```python
from build123d import *

# Parameters (mm, degrees)
SKETCH_R        = 12.5
PAD_DEPTH       = 30
SKETCH001_R     = 5
POCKET_DEPTH    = 10
SKETCH002_R     = 4
POCKET001_DEPTH = 10


with BuildPart() as part:
    # Sketch → Pad (new body)
    with BuildSketch(Plane.XZ):
        Circle(SKETCH_R)
    extrude(amount=PAD_DEPTH)

    # Sketch001 (on Face3 of Pad) → Pocket (cut)
    with BuildSketch(Plane.XZ.offset(30)):
        Circle(SKETCH001_R)
    extrude(amount=-POCKET_DEPTH, mode=Mode.SUBTRACT)

    # Sketch002 (on Face2 of Pocket) → Pocket001 (cut)
    with BuildSketch(Plane(origin=(0, 0, 0), x_dir=(1, 0, 0), z_dir=(0, 1, 0))):
        Circle(SKETCH002_R)
    extrude(amount=-POCKET001_DEPTH, mode=Mode.SUBTRACT)


solid = part.part
```
Model file for the job. Use its own axes, mm. A direction names the side the tool comes from. Coordinates: 2 decimals unless noted, no trailing zeros. Write each loop counter-clockwise with the first axis right and the second up, starting at its lowest first coordinate (ties: lowest second). Pieces come first, ordered by that corner, then holes. Notation, with made-up numbers: (30, 87.25) - (85, 87.25) arc R31 cw to (85, 124.25) - close; hole circle Ø10 at (-11, 31.5). An arc over 180 degrees is marked (long way). One line per item, written item: value. Start each with the question number.
1. Flat gauge pins, fed straight in: pin 1 (1 mm diameter, centred on x = 3, z = -1.5, fed in from +Y); pin 2 (2 mm diameter, centred on x = -5, y = -15, fed in from +Z); pin 3 (2 mm diameter, centred on y = -25, z = -9, fed in from -X). Where does each tip first touch, or does it go through?
2. Probe line 1 (Z direction, x = 0, y = -2.25); line 2 (Z direction, x = 0, y = -24.75); line 3 (X direction, y = -8.25, z = -2.75). List the from-to ranges inside material, lowest first. Write a range as from..to.
3. Slice it at C-C (y = -7.75). Write the cut outline in (x, z).
4. Mould opens along Z. For faces 4 (the cylindrical face through (11.923, -14.79, 3.755)), 5 (the flat face through (-3, 0, 3)), 6 (the flat face through (0, -20, 0)) say: released by +Z, released by -Z, zero draft, split by the parting line, or undercut.
5. Tool access for faces 1 (the cylindrical face through (-0.867, -4.93, 3.905)), 2 (the flat face through (-0.2, -30, -5.4)), 3 (the cylindrical face through (-1.08, -25.07, -4.88)): list every direction of +Z, -Z, +X, -X, +Y, -Y with a clear straight run to the whole face (end or side of a thin tool).
6. Slice it at B-B (x = 0). Write the cut outline in (y, z), plus the area to 3 significant figures.
7. Slice it at D-D (y = -12.5). Write the cut outline in (x, z), plus the area to 3 significant figures.
8. Slice it at A-A (z = 0). Write the cut outline in (x, y).
Answers below:
1. pin 1: stops at y = -10
1. pin 2: stops at z = 11.84
1. pin 3: stops at x = -9.6
2. line 1: z = -12.5..-4, 4..12.5
2. line 2: z = -12.5..-5, 5..12.5
2. line 3: x = -12.19..-2.9, 2.9..12.19
3. outline: circle Ø25 at (0, 0); hole circle Ø8 at (0, 0)
4. face 4: split by the parting line
4. face 5: zero draft
4. face 6: undercut
5. face 1: +Y
5. face 2: +Z, -Z, +X, -X, -Y
5. face 3: -Y
6. outline: (-30, -12.5) - (0, -12.5) - (0, -4) - (-10, -4) - (-10, 4) - (0, 4) - (0, 12.5) - (-30, 12.5) - (-30, 5) - (-20, 5) - (-20, -5) - (-30, -5) - close
6. area: 570 mm^2
7. outline: circle Ø25 at (0, 0)
7. area: 491 mm^2
8. outline: (-12.5, -30) - (-5, -30) - (-5, -20) - (5, -20) - (5, -30) - (12.5, -30) - (12.5, 0) - (4, 0) - (4, -10) - (-4, -10) - (-4, 0) - (-12.5, 0) - close
